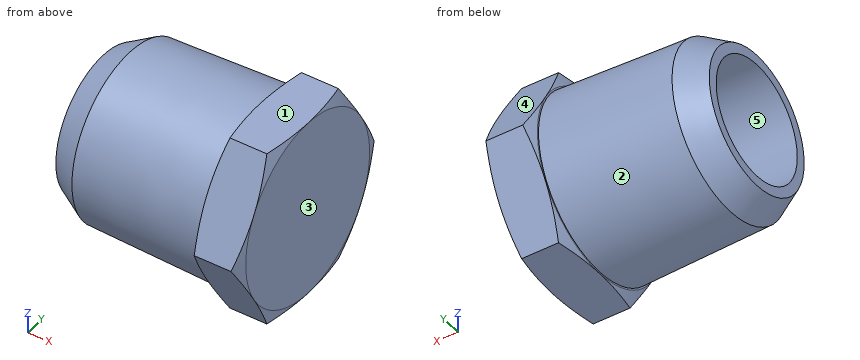
from build123d import *

# Parameters (mm, degrees)
SKETCH2_R          = 8.5725
EXTRUDE1_DEPTH     = 15.25524
EXTRUDE1_DRAFT     = -1.783333333
CHAMFER1_SIZE      = 1.411111111
CHAMFER1_SIZE2     = 2.584686345
EXTRUDE2_DEPTH     = 4.55676
SKETCH4_OUTSIDE_W  = 162.838
SKETCH4_OUTSIDE_H  = 165.54
SKETCH4_OUTSIDE_R  = 8.73125
CUT_EXTRUDE1_DEPTH = 24.882972442
CUT_EXTRUDE1_DRAFT = -70
SKETCH10_OUTSIDE_W = 142.948
SKETCH10_OUTSIDE_H = 145.65
SKETCH10_OUTSIDE_R = 8.73125
CUT_EXTRUDE2_DEPTH = 21.263350565
CUT_EXTRUDE2_DRAFT = -70


with BuildPart() as part:
    # Sketch2 → Extrude1 (with draft: the straight prism first)
    with BuildSketch(Plane(origin=(5.34924, 0, 0), x_dir=(0, 0, -1), z_dir=(1, 0, 0))):
        Circle(SKETCH2_R)
    extrude(amount=-EXTRUDE1_DEPTH)
    # Extrude1: the draft: its side faces are tilted about the plane it starts from
    extrude1_sides = [part.faces().sort_by_distance(p)[0] for p in [
        (-2.27838, 0, 8.5725),
    ]]
    draft(extrude1_sides, Plane(origin=(5.34924, 0, 0), x_dir=(0, 0, -1), z_dir=(1, 0, 0)), EXTRUDE1_DRAFT)

    # Chamfer1
    chamfer1_edges = [part.edges().sort_by_distance(p)[0] for p in [
        (-9.906, 0, 8.097526681),
    ]]
    chamfer1_side = [part.faces().sort_by_distance(p)[0] for p in [
        (-9.906, 0, 0),
    ]]
    chamfer(chamfer1_edges, length=CHAMFER1_SIZE, length2=CHAMFER1_SIZE2, reference=chamfer1_side[0])

    # Sketch3 → Extrude2 (add)
    with BuildSketch(Plane.ZY.offset(-5.34924)):
        Polygon((8.73125, 5.040989538), (0, 10.081979076), (-8.73125, 5.040989538), (-8.73125, -5.040989538), (0, -10.081979076), (8.73125, -5.040989538), align=None)
    extrude(amount=-EXTRUDE2_DEPTH)


with BuildPart() as cut_extrude1_tool:
    # Sketch4 outside → Cut-Extrude1 (with draft: the straight prism first)
    with BuildSketch(Plane(origin=(9.906, 0, 0), x_dir=(0, 0, -1), z_dir=(1, 0, 0))):
        Rectangle(SKETCH4_OUTSIDE_W, SKETCH4_OUTSIDE_H)
        Circle(SKETCH4_OUTSIDE_R, mode=Mode.SUBTRACT)
    extrude(amount=-CUT_EXTRUDE1_DEPTH)
    # Cut-Extrude1: the draft: its side faces are tilted about the plane it starts from
    cut_extrude1_sides = [cut_extrude1_tool.faces().sort_by_distance(p)[0] for p in [
        (-2.535486221, -82.77, 0),
        (-2.535486221, 0, -81.419),
        (-2.535486221, 82.77, 0),
        (-2.535486221, 0, 81.419),
        (-2.535486221, 0, 8.73125),
    ]]
    draft(cut_extrude1_sides, Plane(origin=(9.906, 0, 0), x_dir=(0, 0, -1), z_dir=(1, 0, 0)), CUT_EXTRUDE1_DRAFT)


with BuildPart() as part_1:
    add(part.part)

    # Cut-Extrude1: cut by cut_extrude1_tool
    add(cut_extrude1_tool.part, mode=Mode.SUBTRACT)


with BuildPart() as cut_extrude2_tool:
    # Sketch10 outside → Cut-Extrude2 (with draft: the straight prism first)
    with BuildSketch(Plane.ZY.offset(-5.34924)):
        Rectangle(SKETCH10_OUTSIDE_W, SKETCH10_OUTSIDE_H)
        Circle(SKETCH10_OUTSIDE_R, mode=Mode.SUBTRACT)
    extrude(amount=-CUT_EXTRUDE2_DEPTH)
    # Cut-Extrude2: the draft: its side faces are tilted about the plane it starts from
    cut_extrude2_sides = [cut_extrude2_tool.faces().sort_by_distance(p)[0] for p in [
        (15.980915282, -72.825, 0),
        (15.980915282, 0, 71.474),
        (15.980915282, 72.825, 0),
        (15.980915282, 0, -71.474),
        (15.980915282, 0, -8.73125),
    ]]
    draft(cut_extrude2_sides, Plane.ZY.offset(-5.34924), CUT_EXTRUDE2_DRAFT)


with BuildPart() as part_2:
    add(part_1.part)

    # Cut-Extrude2: cut by cut_extrude2_tool
    add(cut_extrude2_tool.part, mode=Mode.SUBTRACT)

    # Sketch12 → Cut-Revolve1 (revolve, cut)
    with BuildSketch(Plane.XY, mode=Mode.PRIVATE) as cut_revolve1_sk:
        Polygon((-9.906, 0), (6.735918438, 0), (3.302, 5.715), (-9.906, 5.715), align=None)
    revolve(cut_revolve1_sk.sketch.rotate(Axis((6.735918438, 0, 0), (1, 0, 0)), 180), axis=Axis((6.735918438, 0, 0), (1, 0, 0)), mode=Mode.SUBTRACT)


solid = part_2.part
Can you work these out from the model? Positions are in its coordinate system, mm. Face numbers are marked on the shaded views. A direction names the side the tool comes from. Coordinates: 2 decimals unless noted, no trailing zeros. Loops run counter-clockwise (first coordinate to the right, second up) from the corner with the lowest first, then second, coordinate; pieces in that order, holes last. Notation, with made-up numbers: M 8.25,79 L 56.25,79 A31 cw 56.25,112 Z; hole C 5.25,51 d9. An arc over 180 degrees is marked long. Return JSON: item names as keys, results as strings. Group by question number.
Item 1: Thinking about a two-plate mould opening in Z: for the marked faces 3, 4 and 5, which applies, released by +Z, released by -Z, zero draft, split by the parting line, or undercut?
Item 2: I'm going to push flat-ended pins straight in: pin 1 Ø5 at (x, z) = (5.5, 3.5) entering from -Y; pin 2 Ø6 at (x, y) = (-1.5, 2.5) entering from +Z; pin 3 Ø3 at (x, y) = (-5, -8) entering from +Z. Where does each tip first touch, or does it pass through?
Item 3: If I drill on L1, parallel to Z at x = -8.5, y = -0.75; L2, parallel to Y at x = 3, z = -1; L3, parallel to Z at x = -0.25, y = 0 (3 decimals), over which ranges is the centre line in solid material (lowest first)? Write a range as from..to.
Item 4: Imagine slicing it at C-C (x = -1.25). Please give me the cut outline in (y, z) (3 decimals).
Item 5: Imagine slicing it at B-B (x = 8.5). Please give me the cut outline in (y, z).
Item 6: On a 3-axis mill with a long thin cutter (end or side, diameter ignored), from which of +Z, -Z, +X, -X, +Y, -Y can I reach the whole of each face in a straight line? I mean the marked faces 1 and 2. Say none if no direction works.
Item 7: Imagine slicing it at A-A (x = -5.25). Please give me the cut outline in (y, z) (1 decimal).
Verdict:
{
 "1": {"face 3": "zero draft", "face 4": "released by +Z", "face 5": "undercut"},
 "2": {"pin 1": "stops at y = -9.5", "pin 2": "stops at z = 8.42", "pin 3": "stops at z = 5.08"},
 "3": {"L1": "z = -7.46..-5.67, 5.67..7.46", "L2": "y = -8.44..-5.63, 5.63..8.44", "L3": "z = -8.398..-5.715, 5.715..8.398"},
 "4": {"outline": "C 0,0 d16.734; hole C 0,0 d11.43"},
 "5": {"outline": "M -10.08,0 L -5.04,-8.73 L 5.04,-8.73 L 10.08,0 L 5.04,8.73 L -5.04,8.73 Z"},
 "6": {"face 1": "+Z, +X, -X, +Y, -Y", "face 2": "-X"},
 "7": {"outline": "C 0,0 d16.5; hole C 0,0 d11.4"}
}
